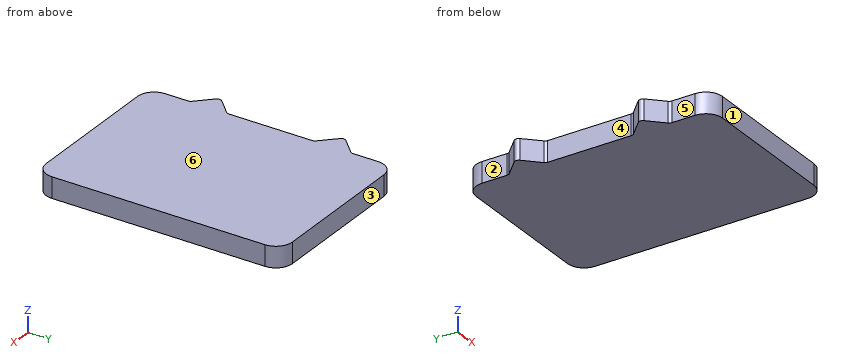
Autodesk Inventor part; units mm, degrees
ref_plane "hal_XY" through (0, 0, 0) normal (0, 0, 1) x (1, 0, 0)
ref_plane "hal_YZ" through (0, 0, 0) normal (1, 0, 0) x (0, 1, 0)
ref_plane "hal_ZX" through (0, 0, 0) normal (0, 1, 0) x (0, 0, 1)
sketch "Sketch_1" plane through (0, 0, 0) normal (0, 0, 1) x (1, 0, 0)
  arc A0 (-5.2586, 3.1414) -> (-5.2586, 2.8586) centre (-5.1172, 3) ccw
  line L0 (-5.2586, 2.8586) -> (-4.5586, 2.1586)
  arc A1 (-4.5, 2.0172) -> (-4.5586, 2.1586) centre (-4.7, 2.0172) ccw
  line L1 (-4.5, 2.0172) -> (-4.5, -2.0172)
  arc A2 (-4.5586, -2.1586) -> (-4.5, -2.0172) centre (-4.7, -2.0172) ccw
  line L2 (-4.5586, -2.1586) -> (-5.2586, -2.8586)
  arc A3 (-5.2586, -2.8586) -> (-5.2586, -3.1414) centre (-5.1172, -3) ccw
  line L3 (-5.2586, -3.1414) -> (-4.5586, -3.8414)
  arc A4 (-4.5, -3.9828) -> (-4.5586, -3.8414) centre (-4.7, -3.9828) ccw
  line L4 (-4.5, -3.9828) -> (-4.5, -5.1)
  arc A5 (-4.5, -5.1) -> (-3.7, -5.9) centre (-3.7, -5.1) ccw
  line L5 (-3.7, -5.9) -> (3, -5.9)
  arc A6 (3, -5.9) -> (3.8, -5.1) centre (3, -5.1) ccw
  line L6 (3.8, -5.1) -> (3.8, 5.2)
  arc A7 (3.8, 5.2) -> (3, 6) centre (3, 5.2) ccw
  line L7 (3, 6) -> (-3.7, 6)
  arc A8 (-3.7, 6) -> (-4.5, 5.2) centre (-3.7, 5.2) ccw
  line L8 (-4.5, 5.2) -> (-4.5, 3.9828)
  arc A9 (-4.5586, 3.8414) -> (-4.5, 3.9828) centre (-4.7, 3.9828) ccw
  line L9 (-4.5586, 3.8414) -> (-5.2586, 3.1414)
extrude "Extrusion1" add sketch "Sketch_1" along normal blind 1
ref_plane "hal_XY" through (0, 0, 0) normal (0, 0, 1) x (1, 0, 0)
ref_plane "hal_YZ" through (0, 0, 0) normal (1, 0, 0) x (0, 1, 0)
ref_plane "hal_ZX" through (0, 0, 0) normal (0, 1, 0) x (0, 0, 1)
ref_plane "s01_XY" through (0, 0, 1) normal (0, 0, 1) x (1, 0, 0)
ref_plane "s01_YZ" through (0, 0, 1) normal (1, 0, 0) x (0, 1, 0)
ref_plane "s01_ZX" through (0, 0, 1) normal (0, 1, 0) x (0, 0, 1)
properties part number "SCHUNK-9962713 Bracket MPG 40"
Work out the finished part from the listing and answer in its coordinate system (mm). Face numbers are marked on the shaded views. A direction names the side the tool comes from. Round coordinates to 2 decimals unless told otherwise and drop trailing zeros. Write each loop counter-clockwise with the first axis right and the second up, starting at its lowest first coordinate (ties: lowest second). Pieces come first, ordered by that corner, then holes. Notation, with made-up numbers: (-26.5, 20) -> (-14.5, 20) arc R24 ccw to (-14.5, 38) -> close; hole circle Ø1 at (3.25, -32.5). An arc over 180 degrees is marked (long way). Write each question's results on one line, items separated by ' | '.
Item 1: Which of the six approach directions +Z, -Z, +X, -X, +Y, -Y give full straight-line access (tool end or side, diameter ignored) to the marked faces 5 and 6?
Result set:
face 5: +Z, -Z, -X, -Y | face 6: +Z, +X, -X, +Y, -Y
Item 2: A cutting plane is placed at C-C, the plane y = 3.5. Determine the outline of the cut face in (x, z), plus the area to 3 significant figures.
Result set:
outline: (-4.9, 0) -> (3.8, 0) -> (3.8, 1) -> (-4.9, 1) -> close | area: 8.70 mm^2
Item 3: A cutting plane is placed at A-A, the plane z = 0.25. Determine the outline of the cut face in (x, y), plus the area to 3 significant figures.
Result set:
outline: (-5.26, -3.14) -> (-4.56, -3.84) arc R0.2 cw to (-4.5, -3.98) -> (-4.5, -5.1) arc R0.8 ccw to (-3.7, -5.9) -> (3, -5.9) arc R0.8 ccw to (3.8, -5.1) -> (3.8, 5.2) arc R0.8 ccw to (3, 6) -> (-3.7, 6) arc R0.8 ccw to (-4.5, 5.2) -> (-4.5, 3.98) arc R0.2 cw to (-4.56, 3.84) -> (-5.26, 3.14) arc R0.2 ccw to (-5.26, 2.86) -> (-4.56, 2.16) arc R0.2 cw to (-4.5, 2.02) -> (-4.5, -2.02) arc R0.2 cw to (-4.56, -2.16) -> (-5.26, -2.86) arc R0.2 ccw to start | area: 99.8 mm^2
Item 4: The mould has two halves that part along Y. Classify the marked faces 1, 2, 3 and 4: +Y half, -Y half, draft (parallel to the pull), parting line (faces both ways), or undercut.
Result set:
face 1: -Y half | face 2: draft | face 3: +Y half | face 4: undercut
Item 5: A cutting plane is placed at B-B, the plane y = -4.75. Determine the outline of the cut face in (x, z).
Result set:
outline: (-4.5, 0) -> (3.8, 0) -> (3.8, 1) -> (-4.5, 1) -> close
Item 6: A flat-ended cylindrical pin translates along its axis: P1, Ø0.5, axis at y = -1, z = 0.5, coming from the -X side. Find the tip coordinate at first contact, or state that the pin passes through.
Result set:
P1: x = -4.5
Item 7: Find the intervals of material crossed by line 1 along X through (y, z) = (-4.75, 0.6); line 2 along Y through (x, z) = (-5, 0.8); line 3 along X through (y, z) = (2.25, 0.85), in increasing order. Write a range as [from, to].
Result set:
line 1: [-4.5, 3.8] | line 2: [-3.4, -2.6], [2.6, 3.4] | line 3: [-4.65, 3.8]
